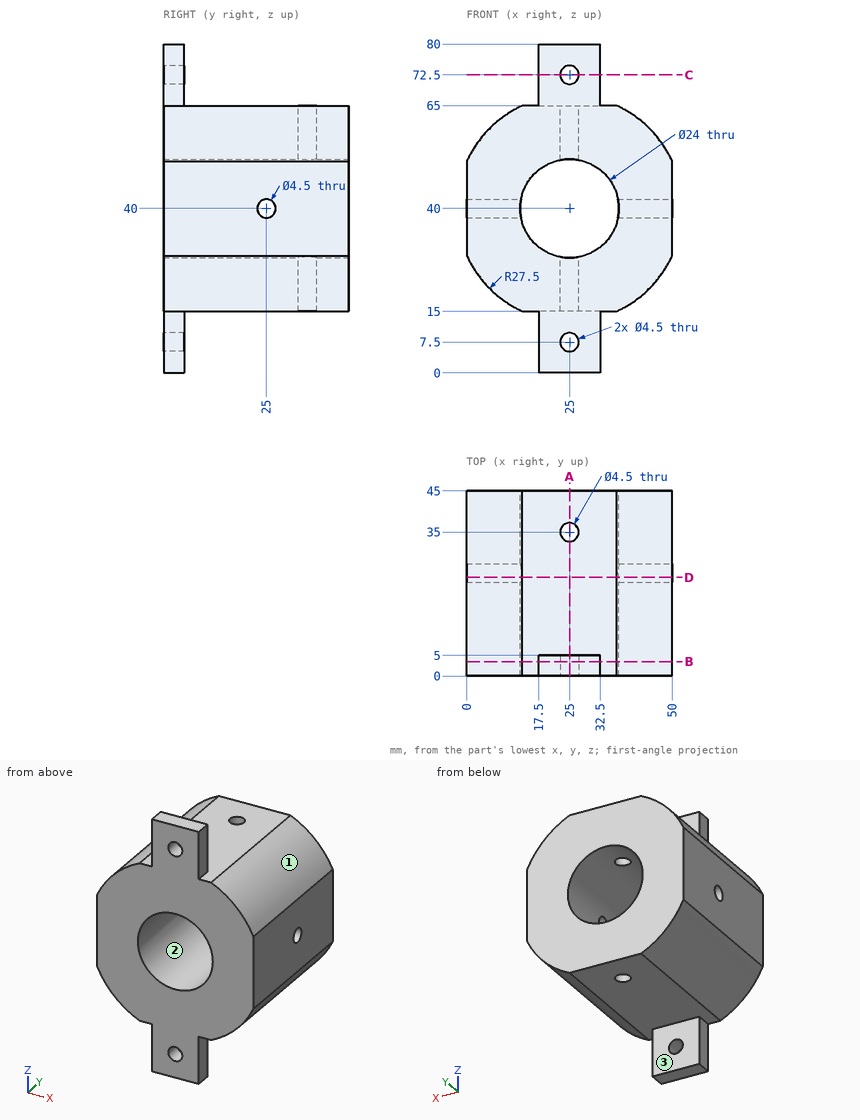
Source: three-view drawing plus pictorial views. Frame: mm from the lowest corner of the part. Round coordinates to 2 decimals unless told otherwise and drop trailing zeros. Loops run counter-clockwise (first coordinate to the right, second up) from the corner with the lowest first, then second, coordinate; pieces in that order, holes last.
Item 1: Section A-A, the plane x = 25. Output: boundary loops of the cut face in (y, z).
Checked values:
outline: (0, 0) - (5, 0) - (5, 5.25) - (0, 5.25) - close; (0, 9.75) - (5, 9.75) - (5, 15) - (32.75, 15) - (32.75, 28) - (0, 28) - close; (0, 52) - (32.75, 52) - (32.75, 65) - (5, 65) - (5, 70.25) - (0, 70.25) - close; (0, 74.75) - (5, 74.75) - (5, 80) - (0, 80) - close; (37.25, 15) - (45, 15) - (45, 28) - (37.25, 28) - close; (37.25, 52) - (45, 52) - (45, 65) - (37.25, 65) - close
Item 2: Section B-B, the plane y = 3.5. Output: boundary loops of the cut face in (x, z), plus the area to 3 significant figures.
Checked values:
outline: (0, 28.54) arc R27.5 ccw to (13.54, 15) - (17.5, 15) - (17.5, 0) - (32.5, 0) - (32.5, 15) - (36.46, 15) arc R27.5 ccw to (50, 28.54) - (50, 51.46) arc R27.5 ccw to (36.46, 65) - (32.5, 65) - (32.5, 80) - (17.5, 80) - (17.5, 65) - (13.54, 65) arc R27.5 ccw to (0, 51.46) - close; hole circle Ø24 at (25, 40); hole circle Ø4.5 at (25, 7.5); hole circle Ø4.5 at (25, 72.5)
area: 2,190 mm2
Item 3: Contact query for flat-ended pins moving along their axis: P1, Ø1, axis at x = 13.5, y = 17, coming from the -Z side; P2, Ø1.5, axis at y = 2, z = 69, coming from the +X side; P3, Ø5.5, axis at y = 2, z = 70, coming from the -X side; P4, Ø25, axis at x = 21.5, y = 17, coming from the +Z side. Output: stop coordinate, or through.
Checked values:
P1: stops at z = 15
P2: stops at x = 32.5
P3: stops at x = 17.5
P4: stops at z = 80
Item 4: Section D-D, the plane y = 24. Output: boundary loops of the cut face in (x, z).
Checked values:
outline: (0, 28.54) arc R27.5 ccw to (13.54, 15) - (36.46, 15) arc R27.5 ccw to (50, 28.54) - (50, 37.98) - (36.83, 37.98) arc R12 cw to (13.17, 37.98) - (0, 37.98) - close; (0, 42.02) - (13.17, 42.02) arc R12 cw to (36.83, 42.02) - (50, 42.02) - (50, 51.46) arc R27.5 ccw to (36.46, 65) - (13.54, 65) arc R27.5 ccw to (0, 51.46) - close
Item 5: Mould query, pull axis X, two halves, no side actions, for the marked faces 1, 2 and 3. Classes: released by +X, released by -X, zero draft, split by the parting line, or undercut.
Checked values:
face 1: released by +X
face 2: undercut
face 3: zero draft
Item 6: Section C-C, the plane z = 72.5. Output: boundary loops of the cut face in (x, y).
Checked values:
outline: (17.5, 0) - (22.75, 0) - (22.75, 5) - (17.5, 5) - close; (27.25, 0) - (32.5, 0) - (32.5, 5) - (27.25, 5) - close
Item 7: Line query: L1, parallel to Z at x = 25, y = 3.5; L2, parallel to Z at x = 25, y = 30; L3, parallel to Y at x = 25, z = 57. Output: solid intervals per line, ascending.
Checked values:
L1: z = 0 to 5.25, 9.75 to 28, 52 to 70.25, 74.75 to 80
L2: z = 15 to 28, 52 to 65
L3: y = 0 to 32.75, 37.25 to 45
